Read the model definition and answer for the solid it produces. Units are mm, in the model's axes. A direction names the side the tool comes from. Round coordinates to 2 decimals unless told otherwise and drop trailing zeros. Order: outer loops, then holes, each group sorted by start corner. A loop starts at its lowest first (then second) coordinate and runs counter-clockwise, first axis right, second up. Notation, with made-up numbers: (79.25, 23.5) -> (136.25, 23.5) arc R15 ccw to (136.25, 45.5) -> close; hole circle Ø9 at (45.5, 21). An arc over 180 degrees is marked (long way). Use a Markdown table: item, result. Add a question column.
1. Given pin 1 (4.5 mm diameter, centred on y = -607, z = 4, fed in from +X); pin 2 (4 mm diameter, centred on x = -43, z = 53, fed in from +Y); pin 3 (8 mm diameter, centred on x = 65, y = -65.5, fed in from +Z); pin 4 (12.5 mm diameter, centred on x = 262, y = -614.5, fed in from +Z), each flat-ended and moving along its own axis, determine where each tip first touches the part or whether it passes through.
2. For faces 1 (the face through (-10, -304, -10)), 2 (the face through (495, -296, -2)), 3 (the face through (249, -612, 15)), 4 (the face through (249, -612, 0)), determine the directions among +Z, -Z, +X, -X, +Y, -Y from which every point of the face is accessible in a straight line to the end or side of a thin tool.
3. Section A-A, the plane z = 42.5 is taken. Give the vertices of the cut face in (x, y).
4. The mould has two halves that part along Y. Classify faces 5 (the face through (-7, 0, 2)), 6 (the face through (-251, -612, 0)), 7 (the face through (-115, -10, 7)): +Y half, -Y half, draft (parallel to the pull), parting line (faces both ways), or undercut.
5. Section B-B, the plane y = -311 is taken. Give the vertices of the cut face in (x, z).
6. Consider L1, parallel to X at y = -122.5, z = 47.5; L2, parallel to Y at x = -18.5, z = 73.5; L3, parallel to Y at x = -311, z = 6. Determine where each line is inside the solid, lowest interval first. Write a range as [from, to].
7. Section D-D, the plane x = -44 is taken. Give the vertices of the cut face in (y, z).
8. Section C-C, the plane x = -187 is taken. Give the vertices of the cut face in (y, z).
```python
from build123d import *

# Parameters (mm, degrees)
F0_W     = 990
F0_H     = 280
F1_DEPTH = 600
F2_T     = -10
F3_W     = 20
F3_H     = 580
F4_DEPTH = 243
F5_W     = 180
F5_H     = 15
F6_DEPTH = 25


with BuildPart() as f1:
    # F0 (on Front) → F1 (new body)
    with BuildSketch(Plane.XZ):
        Rectangle(F0_W, F0_H)
    extrude(amount=F1_DEPTH)

    # F2
    f2_openings = [f1.faces().sort_by_distance(p)[0] for p in [
        (0, -300, 140),
    ]]
    offset(amount=F2_T, openings=f2_openings)

    # F3 (on face) → F4 (join)
    with BuildSketch(Plane.XY.offset(-130)):
        with Locations((0, -300)):
            Rectangle(F3_W, F3_H)
    extrude(amount=F4_DEPTH)

    # F5 (on face) → F6 (join)
    with BuildSketch(Plane.XZ.offset(600)):
        with Locations((250, 7.5)):
            Rectangle(F5_W, F5_H)
        with Locations((-250, 7.5)):
            Rectangle(F5_W, F5_H)
    extrude(amount=F6_DEPTH)


solid = f1.part
```
Verdict:
| question | item | result |
|---|---|---|
| 1 | pin 1 | stops at x = 340 |
| 1 | pin 2 | stops at y = 0 |
| 1 | pin 3 | stops at z = -130 |
| 1 | pin 4 | stops at z = 15 |
| 2 | face 1 | +Z |
| 2 | face 2 | +Z, -Z, +X, +Y, -Y |
| 2 | face 3 | +Z, +X, -X, -Y |
| 2 | face 4 | -Z, +X, -X, -Y |
| 3 | outline | (-495, -600) -> (495, -600) -> (495, 0) -> (-495, 0) -> close; hole (-485, -590) -> (-10, -590) -> (-10, -10) -> (-485, -10) -> close; hole (10, -590) -> (485, -590) -> (485, -10) -> (10, -10) -> close |
| 4 | face 5 | +Y half |
| 4 | face 6 | draft |
| 4 | face 7 | undercut |
| 5 | outline | (-495, -140) -> (495, -140) -> (495, 140) -> (485, 140) -> (485, -130) -> (10, -130) -> (10, 113) -> (-10, 113) -> (-10, -130) -> (-485, -130) -> (-485, 140) -> (-495, 140) -> close |
| 6 | L1 | x = [-495, -485], [-10, 10], [485, 495] |
| 6 | L2 | y = [-600, -590], [-10, 0] |
| 6 | L3 | y = [-625, -590], [-10, 0] |
| 7 | outline | (-600, -140) -> (0, -140) -> (0, 140) -> (-10, 140) -> (-10, -130) -> (-590, -130) -> (-590, 140) -> (-600, 140) -> close |
| 8 | outline | (-625, 0) -> (-600, 0) -> (-600, -140) -> (0, -140) -> (0, 140) -> (-10, 140) -> (-10, -130) -> (-590, -130) -> (-590, 140) -> (-600, 140) -> (-600, 15) -> (-625, 15) -> close |
